```python
from build123d import *

# Parameters (mm, degrees)
BOSS_EXTRUDE1_DEPTH = 90


with BuildPart() as part:
    # Sketch1 → Boss-Extrude1 (new, symmetric)
    with BuildSketch(Plane.XY):
        with BuildLine():
            Line((-20, 22), (-20, -20))
            Line((-20, -20), (22, -20))
            ThreePointArc((22, -20), (24.121320344, -20.878679656), (25, -23))
            Line((25, -23), (25, -25))
            Line((25, -25), (-25, -25))
            Line((-25, -25), (-25, 25))
            Line((-25, 25), (-23, 25))
            ThreePointArc((-23, 25), (-20.878679656, 24.121320344), (-20, 22))
        make_face()
    extrude(amount=BOSS_EXTRUDE1_DEPTH, both=True)


solid = part.part
```
The listing builds one solid part. Answer for the finished solid, in the listing's coordinates (mm). A direction names the side the tool comes from. Give positions to 0.01 mm unless a question says otherwise; leave off trailing zeros. Order: outer loops, then holes, each group sorted by start corner. A loop starts at its lowest first (then second) coordinate and runs counter-clockwise, first axis right, second up.
Item 1: The part is cut by section B-B, the plane x = 12. Give the vertices of the cut face in (y, z), and give its area (3 significant figures).
From the geometry:
outline: (-25, -90) - (-20, -90) - (-20, 90) - (-25, 90) - close
area: 900 mm2
Item 2: Given pin 1 Ø3 at (y, z) = (0.5, 13.5) entering from +X; pin 2 Ø10 at (x, z) = (-8.5, -52.5) entering from +Y, each flat-ended and moving along its own axis, determine where each tip first touches the part or whether it passes through.
From the geometry:
pin 1: stops at x = -20
pin 2: stops at y = -20
Item 3: Find the intervals of material crossed by probe 1 along X at (y, z) = (13, -28.5); probe 2 along X at (y, z) = (-21.5, -5.5), in increasing order.
From the geometry:
probe 1: x = -25 to -20
probe 2: x = -25 to 24.6
Item 4: Which of the six approach directions +Z, -Z, +X, -X, +Y, -Y give full straight-line access (tool end or side, diameter ignored) to faces 1 (the face through (-20, 1, 1)), 2 (the face through (0, -25, 1))?
From the geometry:
face 1: +Z, -Z, +X, +Y
face 2: +Z, -Z, +X, -X, -Y
Item 5: The part is cut by section A-A, the plane z = -14. Give the vertices of the cut face in (x, y).
From the geometry:
outline: (-25, -25) - (25, -25) - (25, -23) arc R3 ccw to (22, -20) - (-20, -20) - (-20, 22) arc R3 ccw to (-23, 25) - (-25, 25) - close
